Could you check a few things on this drawing? It's one solid part, dimensions in mm from its lowest x, y, z. Coordinates: 2 decimals unless noted, no trailing zeros. Loops run counter-clockwise (first coordinate to the right, second up) from the corner with the lowest first, then second, coordinate; pieces in that order, holes last.
1) If I drill on line 1 along X through (y, z) = (0.3, 2.4); line 2 along Z through (x, y) = (13, 0.5); line 3 along X through (y, z) = (0.65, 3.55), over which ranges is the centre line in solid material (lowest first)?
2) Imagine slicing it at C-C on x = 12. Please give me the cut outline in (y, z).
3) Imagine slicing it at D-D on z = 2.5. Please give me the cut outline in (x, y), plus the area to 3 significant figures.
4) Imagine slicing it at B-B on z = 1.3. Please give me the cut outline in (x, y).
5) Will this pin go through, and if not, where does the flat tip stop? P1, Ø0.8, axis at x = 6, y = 0.5, coming from the -Z side.
6) Thinking about a two-plate mould opening in X: for the marked faces 1, 2, 3 and 4, which applies, released by +X, released by -X, zero draft, split by the parting line, or undercut?
7) Imagine slicing it at A-A on y = 0.5. Please give me the cut outline in (x, z).
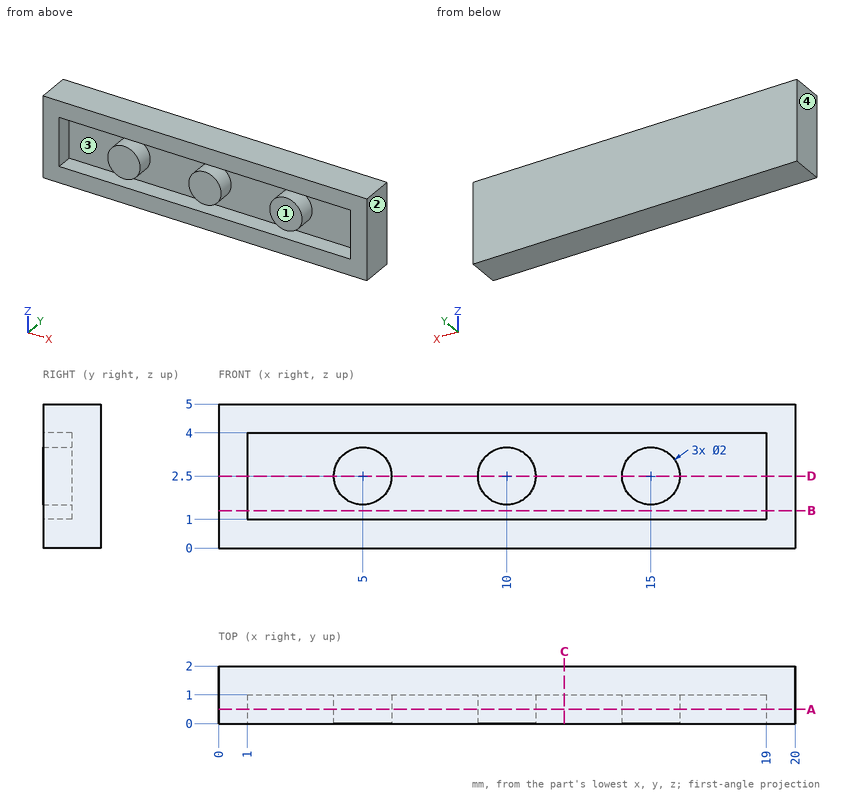
Filled in:
1. line 1: x = 0 to 1, 4.01 to 5.99, 9.01 to 10.99, 14.01 to 15.99, 19 to 20
1. line 2: z = 0 to 1, 4 to 5
1. line 3: x = 0 to 1, 19 to 20
2. outline: (0, 0) - (2, 0) - (2, 5) - (0, 5) - (0, 4) - (1, 4) - (1, 1) - (0, 1) - close
3. outline: (0, 0) - (1, 0) - (1, 1) - (4, 1) - (4, 0) - (6, 0) - (6, 1) - (9, 1) - (9, 0) - (11, 0) - (11, 1) - (14, 1) - (14, 0) - (16, 0) - (16, 1) - (19, 1) - (19, 0) - (20, 0) - (20, 2) - (0, 2) - close
3. area: 28.0 mm2
4. outline: (0, 0) - (1, 0) - (1, 1) - (19, 1) - (19, 0) - (20, 0) - (20, 2) - (0, 2) - close
5. P1: stops at z = 0
6. face 1: zero draft
6. face 2: released by +X
6. face 3: undercut
6. face 4: released by -X
7. outline: (0, 0) - (20, 0) - (20, 5) - (0, 5) - close; circle Ø2 at (5, 2.5); circle Ø2 at (10, 2.5); circle Ø2 at (15, 2.5); hole (1, 1) - (19, 1) - (19, 4) - (1, 4) - close
